from build123d import *

# Parameters (mm, degrees)
ENL_V_MAT_EXTRU_1_DEPTH      = 211.456646367
ENL_V_MAT_EXTRU_1_DEPTH_BACK = 211.456646367
ESQUISSE2_R                  = 8.5
ESQUISSE3_R                  = 90
ENL_V_MAT_EXTRU_2_DEPTH      = 4
ENL_V_START                  = -3
ESQUISSE6_R                  = 65
ENL_V_MAT_EXTRU_5_DEPTH      = 12
ENL_V_MAT_EXTRU_6_DEPTH      = 211.456646367
ENL_V_MAT_EXTRU_6_DEPTH_BACK = 211.456646367
ESQUISSE7_R                  = 60


with BuildPart() as part:
    # Esquisse1 → Révolution1 (revolve)
    with BuildSketch(Plane.XY, mode=Mode.PRIVATE) as r_volution1_sk:
        Polygon((22, 0), (0, 0), (0, 100), (10, 100), (10, 148), (22, 148), align=None)
    revolve(r_volution1_sk.sketch.rotate(Axis((22, 0, 0), (-1, 0, 0)), 90), axis=Axis((22, 0, 0), (-1, 0, 0)))

    # Esquisse2 → Enlèv. mat.-Extru.1 (cut, two sides: drawn at the far end of the back side and taken through both)
    with BuildSketch(Plane(origin=(22, 0, 0), x_dir=(0, 0, -1), z_dir=(1, 0, 0)).offset(-ENL_V_MAT_EXTRU_1_DEPTH_BACK)):
        with Locations((0, 130)):
            Circle(ESQUISSE2_R)
        with Locations((0, -130)):
            Circle(ESQUISSE2_R)
    extrude(amount=ENL_V_MAT_EXTRU_1_DEPTH + ENL_V_MAT_EXTRU_1_DEPTH_BACK, mode=Mode.SUBTRACT)

    # Esquisse3 → Enlèv. mat.-Extru.2 (cut)
    with BuildSketch(Plane(origin=(22, 0, 0), x_dir=(0, 0, -1), z_dir=(1, 0, 0))):
        Circle(ESQUISSE3_R)
    extrude(amount=-ENL_V_MAT_EXTRU_2_DEPTH, mode=Mode.SUBTRACT)

    # Esquisse6 → Enlèv. mat.-Extru.5 (cut)
    with BuildSketch(Plane(origin=(18, 0, 0), x_dir=(0, 0, -1), z_dir=(1, 0, 0)).offset(ENL_V_START)):
        Circle(ESQUISSE6_R)
    extrude(amount=-ENL_V_MAT_EXTRU_5_DEPTH, mode=Mode.SUBTRACT)

    # Esquisse7 → Enlèv. mat.-Extru.6 (cut, two sides: drawn at the far end of the back side and taken through both)
    with BuildSketch(Plane(origin=(22, 0, 0), x_dir=(0, 0, -1), z_dir=(1, 0, 0)).offset(-ENL_V_MAT_EXTRU_6_DEPTH_BACK)):
        Circle(ESQUISSE7_R)
    extrude(amount=ENL_V_MAT_EXTRU_6_DEPTH + ENL_V_MAT_EXTRU_6_DEPTH_BACK, mode=Mode.SUBTRACT)


solid = part.part
Verification items for the finished model (mm, model axes). A direction names the side the tool comes from. Round coordinates to 2 decimals unless told otherwise and drop trailing zeros. Loops run counter-clockwise (first coordinate to the right, second up) from the corner with the lowest first, then second, coordinate; pieces in that order, holes last. Notation, with made-up numbers: (74, 51.5) - (91, 51.5) arc R24 ccw to (91, 86.5) - close; hole circle Ø10 at (-24.75, 40). An arc over 180 degrees is marked (long way). Answer in a Markdown table with one row per item. Add a question column.
Q1. Tool access check on faces 5 (the face through (18, -19, -59)), 6 (the face through (15, -57.5, -19)), 7 (the face through (16.48, 2.64, 59.94)), 8 (the face through (5.07, -30.04, -95.38)), 9 (the face through (0, 43, 43)). Record the directions out of +Z, -Z, +X, -X, +Y, -Y that give a thin tool (end or side, any length) a straight path to the whole face; none if there is none.
Q2. Material ranges on line 1 (Y direction, x = 18.25, z = 0); line 2 (X direction, y = 40, z = 50); line 3 (X direction, y = 0.5, z = -80.5), recorded low to high.
Q3. Gauge pin test, flat ends, axial feed: pin 1 (6 mm diameter, centred on x = 14.5, y = -29, fed in from -Z); pin 2 (1.5 mm diameter, centred on x = 6.5, z = 2, fed in from +Y); pin 3 (2 mm diameter, centred on x = 15.5, z = -104.5, fed in from -Y). Record the tip position at first contact, or that the pin passes through.
Q4. Section check C-C on z = 84. Enter the section's corners in (x, y).
Q5. Section check D-D on y = 130. Enter the section's corners in (x, z).
Q6. Section check B-B on z = 0. State how many separate pieces and enclosed holes the cut face has, plus the area to 3 significant figures.
Q7. Release check for a two-part mould opening along X. For faces 1 (the face through (9.08, 19.52, -62)), 2 (the face through (1.48, 2.64, 59.94)), 3 (the face through (22, 64, -64)), 4 (the face through (10, 97, 31)) record: pulls with the +X half, pulls with the -X half, needs draft (parallel to the pull), parting line crosses it, or undercut.
Q8. Section check A-A on y = 0. Enter the section's corners in (x, z), plus the area to 3 significant figures.
Found:
| question | item | result |
|---|---|---|
| 1 | face 5 | +X |
| 1 | face 6 | none |
| 1 | face 7 | +X, -X |
| 1 | face 8 | -X |
| 1 | face 9 | +Z, -Z, -X, +Y, -Y |
| 2 | line 1 | y = -148 to -138.5, -121.5 to -90, 90 to 121.5, 138.5 to 148 |
| 2 | line 2 | x = 0 to 3, 15 to 18 |
| 2 | line 3 | x = 0 to 18 |
| 3 | pin 1 | stops at z = -145.7 |
| 3 | pin 2 | stops at y = 99.99 |
| 3 | pin 3 | stops at y = -105.79 |
| 4 | outline | (0, -54.26) - (10, -54.26) - (10, -121.85) - (22, -121.85) - (22, -32.31) - (18, -32.31) - (18, 32.31) - (22, 32.31) - (22, 121.85) - (10, 121.85) - (10, 54.26) - (0, 54.26) - close |
| 5 | outline | (10, -70.74) - (22, -70.74) - (22, -8.5) - (10, -8.5) - close; (10, 8.5) - (22, 8.5) - (22, 70.74) - (10, 70.74) - close |
| 6 | separate pieces | 4 |
| 6 | enclosed holes | 0 |
| 6 | area | 2,140 mm² |
| 7 | face 1 | undercut |
| 7 | face 2 | needs draft |
| 7 | face 3 | pulls with the +X half |
| 7 | face 4 | pulls with the -X half |
| 8 | outline | (0, -100) - (10, -100) - (10, -148) - (22, -148) - (22, -90) - (18, -90) - (18, -60) - (15, -60) - (15, -65) - (3, -65) - (3, -60) - (0, -60) - close; (0, 60) - (3, 60) - (3, 65) - (15, 65) - (15, 60) - (18, 60) - (18, 90) - (22, 90) - (22, 148) - (10, 148) - (10, 100) - (0, 100) - close |
| 8 | area | 2,550 mm² |
